Read the model definition and answer for the solid it produces. Units are mm, in the model's axes. Face numbers are marked on the shaded views. Round coordinates to 2 decimals unless told otherwise and drop trailing zeros.
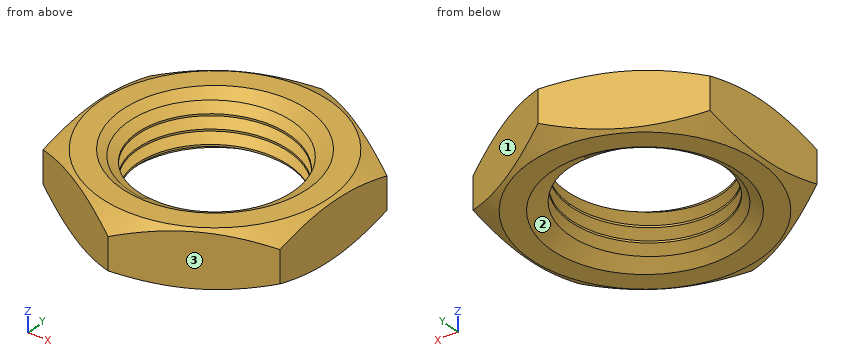
from build123d import *

# Parameters (mm, degrees)
SKETCH_1_W          = 4
SKETCH_1_H          = 5.45
SKETCH_2_R          = 11
CUT_EXTRUDE_1_DEPTH = 16.72021
SKETCH_3_W          = 6
SKETCH_3_H          = 8.964102
SWEEP_1_PITCH       = 1
SWEEP_1_HEIGHT      = 10
SWEEP_1_RADIUS      = 6.05
SWEEP_1_START_ANGLE = 180


with BuildPart() as part:
    # Эскиз1 → Повернуть1 (revolve)
    with BuildSketch(Plane(origin=(0, 0, 0), x_dir=(0, 0, -1), z_dir=(1, 0, 0)), mode=Mode.PRIVATE) as revolve_1_sk:
        with Locations((2, 8.025)):
            Rectangle(SKETCH_1_W, SKETCH_1_H)
    revolve(revolve_1_sk.sketch.rotate(Axis((0, 0, 0), (0, 0, -1)), 90), axis=Axis((0, 0, 0), (0, 0, -1)))

    # Эскиз2 → Вырез-Вытянуть1 (cut, through all)
    with BuildSketch(Plane.XY):
        Circle(SKETCH_2_R)
        Polygon((8.25, -4.76314), (8.25, 4.76314), (0, 9.526279), (-8.25, 4.76314), (-8.25, -4.76314), (0, -9.526279), align=None, mode=Mode.SUBTRACT)
    extrude(amount=-CUT_EXTRUDE_1_DEPTH, mode=Mode.SUBTRACT)

    # Эскиз3 → Вырез-Повернуть1 (revolve, cut)
    with BuildSketch(Plane(origin=(0, 0, 0), x_dir=(0, 0, -1), z_dir=(1, 0, 0)), mode=Mode.PRIVATE) as cut_revolve_1_sk:
        with Locations((2, 6.517949)):
            Rectangle(SKETCH_3_W, SKETCH_3_H)
        Polygon((2, 3.035898), (4, 6.5), (4, 8), (2.845299, 10), (1.154701, 10), (0, 8), (0, 6.5), align=None, mode=Mode.SUBTRACT)
    revolve(cut_revolve_1_sk.sketch.rotate(Axis((0, 0, 0), (0, 0, -1)), 240), axis=Axis((0, 0, 0), (0, 0, -1)), mode=Mode.SUBTRACT)

    # Вырез-По траектории1: sweep along a helix
    with BuildLine() as sweep_1_path:
        add(Helix(SWEEP_1_PITCH, SWEEP_1_HEIGHT, SWEEP_1_RADIUS, center=(0, 0, -4), direction=(0, 0, 1), mode=Mode.PRIVATE).rotate(Axis((0, 0, -4), (0, 0, 1)), SWEEP_1_START_ANGLE))
    with BuildLine() as sweep_1_axis:
        Line((0, 0, -4), (0, 0, 6))
    # Эскиз5 → Вырез-По траектории1 (sweep, cut)
    with BuildSketch(Plane(origin=(-6.05, 0, -4), x_dir=(-1, 0, 0), z_dir=(0, -0.9996541608311538, 0.026297504310521795))):
        Polygon((-0.861695, 0.9975), (0, 0.5), (-0.861695, 0.0025), align=None)
    sweep(path=sweep_1_path.line, binormal=sweep_1_axis.edges()[0], mode=Mode.SUBTRACT)


solid = part.part
Q1. A flat-ended cylindrical pin translates along its axis: pin 1 (1.5 mm diameter, centred on x = -4.5, z = -2.5, fed in from -Y). Find the tip coordinate at first contact, or state that the pin passes through.
Outcome:
pin 1: stops at y = -7.36
Q2. For a pull along Y with two mould halves and no side action, classify the marked faces 1, 2 and 3 as released by +Y, released by -Y, zero draft, split by the parting line, or undercut.
Outcome:
face 1: released by +Y
face 2: undercut
face 3: released by -Y
Q3. Straight lines are drawn through the part: probe 1 along Z at (x, y) = (3.75, -4.5); probe 2 along Z at (x, y) = (4.25, -4); probe 3 along Y at (x, z) = (-2, -3.1). For each, find the intervals that lie inside material, in ascending order.
Outcome:
probe 1: z = -3.63 to -3.25, -3.03 to -2.25, -2.03 to -1.25, -1.03 to -0.37
probe 2: z = -3.62 to -3.24, -3 to -2.24, -2 to -1.24, -1 to -0.38
probe 3: y = -8.37 to -5.33, 4.95 to 8.37
